Part model, mm, in its own coordinate system. Face numbers are marked on the shaded views. A direction names the side the tool comes from. Round coordinates to 2 decimals unless told otherwise and drop trailing zeros. Order: outer loops, then holes, each group sorted by start corner. A loop starts at its lowest first (then second) coordinate and runs counter-clockwise, first axis right, second up. Notation, with made-up numbers: (65, 44) -> (73, 44) arc R22 ccw to (73, 67) -> close; hole circle Ø2 at (38.5, 26.5). An arc over 180 degrees is marked (long way). Answer as a JSON object with one key per item and string values. Group by question number.
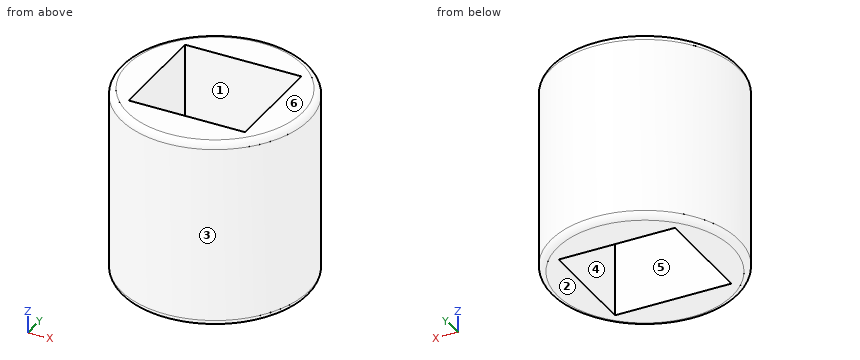
```python
from build123d import *

# Parameters (mm, degrees)
F0_R     = 75.547146
F1_DEPTH = 152.4
F2_R     = 5.08
F3_W     = 93.511396
F3_H     = 86.312428
F4_DEPTH = 152.4
F5_R     = 5.08


with BuildPart() as f1:
    # F0 (on Top) → F1 (new body)
    with BuildSketch(Plane.XY):
        Circle(F0_R)
    extrude(amount=F1_DEPTH)

    # F2
    f2_edges = [f1.edges().sort_by_distance(p)[0] for p in [
        (-75.547146, 0, 152.4),
    ]]
    fillet(f2_edges, radius=F2_R)

    # F3 (on face) → F4 (cut)
    with BuildSketch(Plane.XY.offset(152.4)):
        Rectangle(F3_W, F3_H)
    extrude(amount=-F4_DEPTH, mode=Mode.SUBTRACT)

    # F5
    f5_edges = [f1.edges().sort_by_distance(p)[0] for p in [
        (-75.547146, 0, 0),
    ]]
    fillet(f5_edges, radius=F5_R)


solid = f1.part
```
Q1. Drop flat-ended pins along their axis: pin 1 Ø4 at (y, z) = (-48.5, 20) entering from +X; pin 2 Ø10 at (x, y) = (9.5, -57) entering from -Z; pin 3 Ø10 at (x, z) = (57.5, 88.5) entering from -Y; pin 4 Ø10 at (y, z) = (17.5, 58.5) entering from +X. Give the stop position or say it passes through.
Q2. Band-saw the part on C-C (z = 142). List the corners of the cut face in (x, y), plus the area to 3 significant figures.
Q3. Band-saw the part on A-A (y = 0). List the corners of the cut face in (x, z), plus the area to 3 significant figures.
Q4. Which spindle directions (+Z, -Z, +X, -X, +Y, -Y) get a long thin tool onto all of the face, cutting with end or side? Do the marked faces 1 and 2. Say none if no direction does.
Q5. Two-plate mould, pull along Y, no slides. Class the marked faces 3, 4, 5 and 6: +Y half, -Y half, draft (parallel to the pull), parting line (faces both ways), or undercut.
Q6. Band-saw the part on B-B (x = 0). List the corners of the cut face in (y, z), plus the area to 3 significant figures.
Q7. Wall check: line 1 (Z direction, x = 18.5, y = 68.5); line 2 (Y direction, x = 43.5, z = 13.5); line 3 (X direction, y = 17.5, z = 114). Give the ranges that are in metal, low to high. Write a range as [from, to].
Completed:
{
 "1": {"pin 1": "x = 59.54", "pin 2": "z = 0", "pin 3": "y = -54.32", "pin 4": "x = 74.51"},
 "2": {"outline": "circle Ø151.09 at (0, 0); hole (-46.76, -43.16) -> (46.76, -43.16) -> (46.76, 43.16) -> (-46.76, 43.16) -> close", "area": "9,860 mm2"},
 "3": {"outline": "(-75.55, 5.08) arc R5.08 ccw to (-70.47, 0) -> (-46.76, 0) -> (-46.76, 152.4) -> (-70.47, 152.4) arc R5.08 ccw to (-75.55, 147.32) -> close; (46.76, 0) -> (70.47, 0) arc R5.08 ccw to (75.55, 5.08) -> (75.55, 147.32) arc R5.08 ccw to (70.47, 152.4) -> (46.76, 152.4) -> close", "area": "8,750 mm2"},
 "4": {"face 1": "+Z, -Z", "face 2": "-Z, +X, -X, +Y, -Y"},
 "5": {"face 3": "parting line", "face 4": "undercut", "face 5": "undercut", "face 6": "draft"},
 "6": {"outline": "(-75.55, 5.08) arc R5.08 ccw to (-70.47, 0) -> (-43.16, 0) -> (-43.16, 152.4) -> (-70.47, 152.4) arc R5.08 ccw to (-75.55, 147.32) -> close; (43.16, 0) -> (70.47, 0) arc R5.08 ccw to (75.55, 5.08) -> (75.55, 147.32) arc R5.08 ccw to (70.47, 152.4) -> (43.16, 152.4) -> close", "area": "9,850 mm2"},
 "7": {"line 1": "[0.02, 152.38]", "line 2": "[-61.77, -43.16], [43.16, 61.77]", "line 3": "[-73.49, -46.76], [46.76, 73.49]"}
}
